from build123d import *

# Parameters (mm, degrees)
SKETCH3_W               = 25.4
SKETCH3_H               = 3.175
CUT_EXTRUDE1_DEPTH      = 725.790680128
CUT_EXTRUDE1_DEPTH_BACK = 725.790680128


with BuildPart() as part:
    # Sketch2 → Revolve1 (revolve)
    with BuildSketch(Plane(origin=(0, 0, 0), x_dir=(1, 0, 0), z_dir=(0, 1, 0)), mode=Mode.PRIVATE) as revolve1_sk:
        Polygon((-723.9, 0), (0, 0), (0, 19.05), (12.7, 19.05), (12.7, 25.4), (-19.05, 25.4), (-19.05, 12.7), (-647.7, 12.7), (-647.7, 9.525), (-723.9, 9.525), align=None)
    revolve(revolve1_sk.sketch.rotate(Axis((-723.9, 0, 0), (1, 0, 0)), 180), axis=Axis((-723.9, 0, 0), (1, 0, 0)))

    # Sketch3 → Cut-Extrude1 (cut, two sides)
    with BuildSketch(Plane(origin=(0, 0, 0), x_dir=(1, 0, 0), z_dir=(0, 1, 0))) as cut_extrude1_sk:
        with Locations((-411.48, 11.1125)):
            Rectangle(SKETCH3_W, SKETCH3_H)
    extrude(amount=CUT_EXTRUDE1_DEPTH, mode=Mode.SUBTRACT)
    extrude(cut_extrude1_sk.sketch, amount=-CUT_EXTRUDE1_DEPTH_BACK, mode=Mode.SUBTRACT)


solid = part.part
Build history of the part. All positions in model axes, mm. A direction names the side the tool comes from. Round coordinates to 2 decimals unless told otherwise and drop trailing zeros. Write each loop counter-clockwise with the first axis right and the second up, starting at its lowest first coordinate (ties: lowest second). Pieces come first, ordered by that corner, then holes. Notation, with made-up numbers: (36, 77) -> (78, 77) arc R11 ccw to (78, 94) -> close; hole circle Ø3 at (65.25, -13). An arc over 180 degrees is marked (long way). Use one line per item in the form item = value.
Q1. Band-saw the part on A-A, the plane z = 0. Write the cut outline in (x, y) (3 decimals), then the cut area to 3 significant figures.
Conclusion:
outline = (-723.9, -9.525) -> (-647.7, -9.525) -> (-647.7, -12.7) -> (-19.05, -12.7) -> (-19.05, -25.4) -> (12.7, -25.4) -> (12.7, -19.05) -> (0, -19.05) -> (0, 19.05) -> (12.7, 19.05) -> (12.7, 25.4) -> (-19.05, 25.4) -> (-19.05, 12.7) -> (-647.7, 12.7) -> (-647.7, 9.525) -> (-723.9, 9.525) -> close
area = 18,500 mm²
Q2. Drop flat-ended pins along their axis: P1, Ø3, axis at x = -103.5, z = -2.5, coming from the +Y side; P2, Ø2, axis at x = -66, z = 14.5, coming from the +Y side; P3, Ø12, axis at x = -410, y = 1.5, coming from the +Z side; P4, Ø5, axis at x = -408, y = -3, coming from the -Z side (3 decimals). Give the stop position or say it passes through.
Conclusion:
P1 = 12.66
P2 = through
P3 = 12.7
P4 = -9.525
Q3. Drill centre lines: L1, parallel to Y at x = 4, z = 0; L2, parallel to X at y = -17, z = 13; L3, parallel to Z at x = -210, y = -1. Where is each one in solid material? Low to high.
Conclusion:
L1 = -25.4 to -19.05, 19.05 to 25.4
L2 = -19.05 to 12.7
L3 = -12.66 to 12.66
Q4. Tool access for faces 5 (the cylindrical face through (6.439, 18.597, -4.13)), 6 (the cylindrical face through (-686.33, 9.3, -2.06)), 7 (the flat face through (12.7, -19, -4)): list every direction of +Z, -Z, +X, -X, +Y, -Y with a clear straight run to the whole face (end or side of a thin tool).
Conclusion:
face_5 = +X
face_6 = -X
face_7 = +Z, -Z, +X, +Y, -Y
Q5. Band-saw the part on C-C, the plane x = -134. Write the cut outline in (y, z).
Conclusion:
outline = circle Ø25.4 at (0, 0)
Q6. Band-saw the part on B-B, the plane y = 0. Write the cut outline in (x, z) (3 decimals).
Conclusion:
outline = (-723.9, -9.525) -> (-647.7, -9.525) -> (-647.7, -12.7) -> (-424.18, -12.7) -> (-424.18, -9.525) -> (-398.78, -9.525) -> (-398.78, -12.7) -> (-19.05, -12.7) -> (-19.05, -25.4) -> (12.7, -25.4) -> (12.7, -19.05) -> (0, -19.05) -> (0, 19.05) -> (12.7, 19.05) -> (12.7, 25.4) -> (-19.05, 25.4) -> (-19.05, 12.7) -> (-647.7, 12.7) -> (-647.7, 9.525) -> (-723.9, 9.525) -> close
Q7. Two-plate mould, pull along Z, no slides. Class faces 1 (the cylindrical face through (-3.397, 22.534, 11.721)), 2 (the flat face through (-412, 0, -9.525)), 3 (the flat face through (0, 0, 0)), 4 (the flat face through (-647.7, -9, 5)): released by +Z, released by -Z, zero draft, split by the parting line, or undercut.
Conclusion:
face_1 = split by the parting line
face_2 = released by -Z
face_3 = undercut
face_4 = zero draft
